Source: CAD feature listing. Evaluate the final solid. Frame: model axes, mm. A direction names the side the tool comes from. Coordinates: 2 decimals unless noted, no trailing zeros. Order: outer loops, then holes, each group sorted by start corner. A loop starts at its lowest first (then second) coordinate and runs counter-clockwise, first axis right, second up. Notation, with made-up numbers: (88.25, 67) - (109.25, 67) arc R17 ccw to (109.25, 94) - close; hole circle Ø10 at (-8, -28.75). An arc over 180 degrees is marked (long way). One line per question, with ' | ' between items. Start each with the question number.
(1) Line query: line 1 along Y through (x, z) = (1.5, 0.95); line 2 along Y through (x, z) = (27.5, 0.3); line 3 along X through (y, z) = (-0.5, 1.3). Output: solid intervals per line, ascending.
(2) Contact query for flat-ended pins moving along their axis: P1, Ø1, axis at y = 6.5, z = 1.5, coming from the +X side; P2, Ø0.5, axis at y = -1, z = 1.5, coming from the +X side; P3, Ø1, axis at y = 5, z = 2, coming from the +X side. Output: stop coordinate, or through.
(3) Access query for faces 1 (the flat face through (36, -3, 1)), 2 (the flat face through (0, -1, 1)), 3 (the flat face through (6, 3, 1)). Directions: +Z, -Z, +X, -X, +Y, -Y. A direction counts if a zero-diameter tool reaches every point of the face in a straight line with its end or side. Return the directions, or none.
(4) Section A-A (x = 21). Return the cut outline in (y, z), then the cut area to 3 significant figures.
(5) Section D-D (y = 3.5). Return the cut outline in (x, z).
(6) Section C-C (x = 26). Return the cut outline in (y, z), then the cut area to 3 significant figures.
(7) Section B-B (z = 1.6). Return the cut outline in (x, y), then the cut area to 3 significant figures.
from build123d import *

# Parameters (mm, degrees)
SALIENTE_EXTRUIR1_DEPTH = 2


with BuildPart() as part:
    # Croquis1 → Saliente-Extruir1 (new body)
    with BuildSketch(Plane.XY):
        with BuildLine():
            Line((36, 0), (0, 0))
            Line((0, 0), (0, -1.8))
            Line((0, -1.8), (36, -1.8))
            Line((36, -1.8), (36, -3.8))
            Line((36, -3.8), (0, -3.8))
            ThreePointArc((0, -3.8), (-3.4, -0.4), (0, 3))
            Line((0, 3), (11.23589803, 3))
            ThreePointArc((11.23589803, 3), (17.108100225, 3.881494792), (22.462670855, 6.448275862))
            ThreePointArc((22.462670855, 6.448275862), (30.324267127, 7.550230244), (36, 2))
            Line((36, 2), (36, 0))
        make_face()
    extrude(amount=SALIENTE_EXTRUIR1_DEPTH)


solid = part.part
Response values:
1) line 1: y = -3.8 to -1.8, 0 to 3 | line 2: y = -3.8 to -1.8, 0 to 8 | line 3: x = -3.4 to 0
2) P1: stops at x = 33.17 | P2: stops at x = 0 | P3: stops at x = 34.64
3) face 1: +Z, -Z, +X, +Y, -Y | face 2: +Z, -Z, +X | face 3: +Z, -Z, -X, +Y
4) outline: (-3.8, 0) - (-1.8, 0) - (-1.8, 2) - (-3.8, 2) - close; (0, 0) - (5.55, 0) - (5.55, 2) - (0, 2) - close | area: 15.1 mm²
5) outline: (15.68, 0) - (35.31, 0) - (35.31, 2) - (15.68, 2) - close
6) outline: (-3.8, 0) - (-1.8, 0) - (-1.8, 2) - (-3.8, 2) - close; (0, 0) - (7.87, 0) - (7.87, 2) - (0, 2) - close | area: 19.7 mm²
7) outline: (0, -3.8) - (36, -3.8) - (36, -1.8) - (0, -1.8) - (0, 0) - (36, 0) - (36, 2) arc R9 ccw to (22.46, 6.45) arc R20 cw to (11.24, 3) - (0, 3) arc R3.4 ccw to start | area: 262 mm²
